Answer from the drawing. Dimensions are ordinates in mm from the lowest x, y and z of the part. A direction names the side the tool comes from. Give positions to 0.01 mm unless a question says otherwise; leave off trailing zeros. Loops run counter-clockwise (first coordinate to the right, second up) from the corner with the lowest first, then second, coordinate; pieces in that order, holes last.
Item 1: Section D-D, the plane z = 1.55 is taken. Give the vertices of the cut face in (x, y), and give its area (4 significant figures).
Item 2: Consider line 1 along X through (y, z) = (6.25, 0.45); line 2 along Y through (x, z) = (5, 2.35); line 3 along Y through (x, z) = (11.5, 0.3). Determine where each line is inside the solid, lowest interval first.
Item 3: A tool of negligible diameter and unlimited length cuts with its end or side. For the marked faces 1 and 2, from which of +Z, -Z, +X, -X, +Y, -Y can it reach the whole face along a straight path? Write none if from no direction.
Item 4: Section C-C, the plane x = 9.5 is taken. Give the vertices of the cut face in (y, z), and give its area (3 significant figures).
Item 5: Section B-B, the plane y = 9.25 is taken. Give the vertices of the cut face in (x, z), and give its area (4 significant figures).
Item 6: Each of these flat-tipped pins is pushed along its axis until it touches: pin 1 Ø0.6 at (y, z) = (6, 1.5) entering from -X; pin 2 Ø0.8 at (x, z) = (5.5, 2.5) entering from +Y; pin 3 Ø4 at (x, y) = (4, 12.5) entering from -Z. Where does it stop, or does it pass through?
Item 7: Section A-A, the plane z = 2.4 is taken. Give the vertices of the cut face in (x, y).
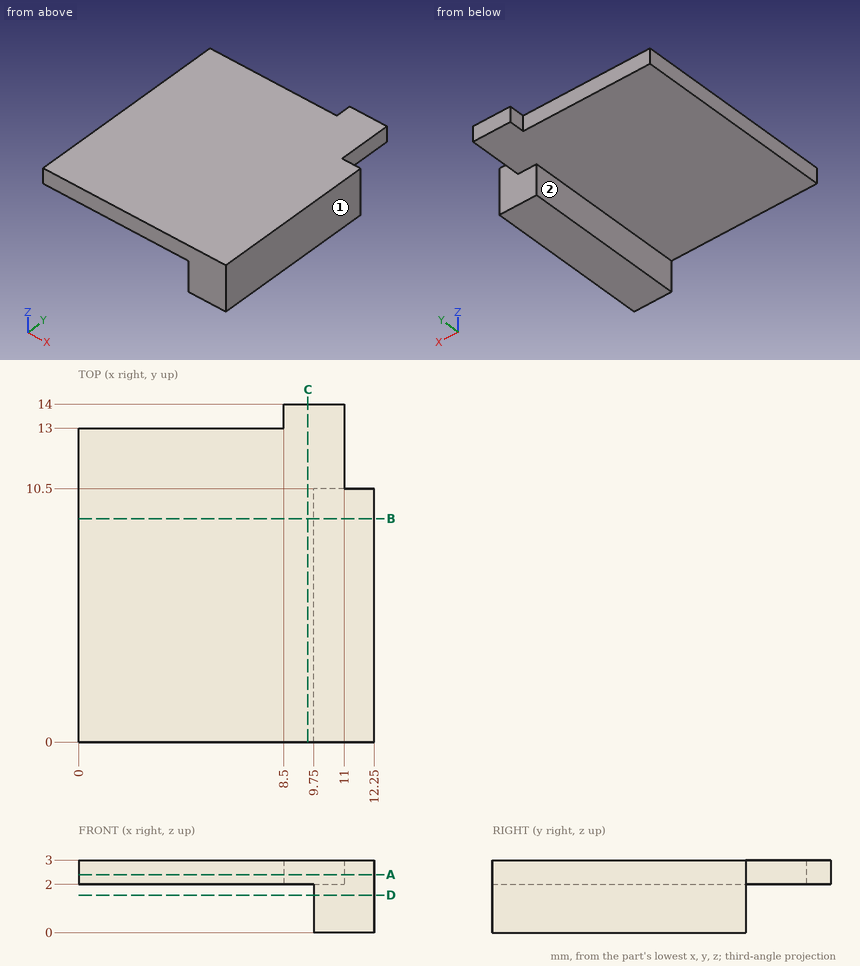
Worked answers:
1. outline: (9.75, 0) - (12.25, 0) - (12.25, 10.5) - (9.75, 10.5) - close
1. area: 26.25 mm2
2. line 1: x = 9.75 to 12.25
2. line 2: y = 0 to 13
2. line 3: y = 0 to 10.5
3. face 1: +Z, -Z, +X, +Y, -Y
3. face 2: -Z, -X, +Y, -Y
4. outline: (0, 2) - (14, 2) - (14, 3) - (0, 3) - close
4. area: 14.0 mm2
5. outline: (0, 2) - (9.75, 2) - (9.75, 0) - (12.25, 0) - (12.25, 3) - (0, 3) - close
5. area: 17.25 mm2
6. pin 1: stops at x = 9.75
6. pin 2: stops at y = 13
6. pin 3: stops at z = 2
7. outline: (0, 0) - (12.25, 0) - (12.25, 10.5) - (11, 10.5) - (11, 14) - (8.5, 14) - (8.5, 13) - (0, 13) - close
